Source: CAD feature listing. Evaluate the final solid. Frame: model axes, mm. Face numbers are marked on the shaded views. A direction names the side the tool comes from. Give positions to 0.01 mm unless a question says otherwise; leave off trailing zeros. Order: outer loops, then holes, each group sorted by start corner. A loop starts at its lowest first (then second) coordinate and runs counter-clockwise, first axis right, second up.
1) Section A-A, the plane z = 4.5. Return loops of the section in (x, y), plus the area to 3 significant figures.
2) Section D-D, the plane y = 30. Return loops of the section in (x, z), plus the area to 4 significant figures.
3) Section C-C, the plane x = -8. Return loops of the section in (y, z), plus the area to 3 significant figures.
4) Access query for the marked faces 1 and 2. Directions: +Z, -Z, +X, -X, +Y, -Y. A direction counts if a zero-diameter tool reaches every point of the face in a straight line with its end or side. Return the directions, or none.
5) Material intervals for line 1 (Y direction, x = 1, z = 0.25); line 2 (X direction, y = 25.5, z = -6.25); line 3 (Y direction, x = -7.75, z = 6.25), sorted ascending.
6) Draft query along Z for the marked faces 3, 4 and 5. Return one class per face: released by +Z, released by -Z, zero draft, split by the parting line, or undercut.
7) Section B-B, the plane x = 0.25. Return loops of the section in (y, z), plus the area to 3 significant figures.
8) First-contact query: P1, Ø2, axis at x = 0.5, z = -3.5, coming from the +Y side; P2, Ø13, axis at x = 3.5, y = 35, coming from the +Z side; P3, Ø2, axis at x = 4.5, z = 2, coming from the +Y side. Flat tips, straight axial feed; report the tip coordinate or a pass-through.
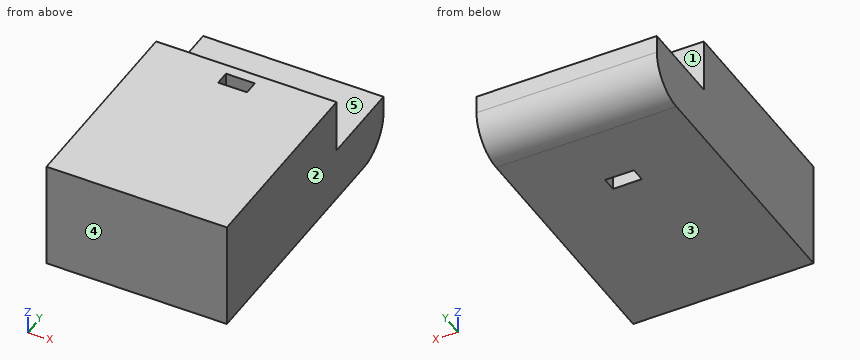
```python
from build123d import *

# Parameters (mm, degrees)
SKIZZE1_W                       = 25
SKIZZE1_H                       = 15
AUFSATZ_LINEAR_AUSTRAGEN1_DEPTH = 40
SKIZZE2_W                       = 25
SKIZZE2_H                       = 7.5
SCHNITT_LINEAR_AUSTRAGEN1_DEPTH = 12
VERRUNDUNG1_R                   = 5
SKIZZE3_W                       = 4
SKIZZE3_H                       = 2
SCHNITT_LINEAR_AUSTRAGEN2_DEPTH = 45.511234537


with BuildPart() as part:
    # Skizze1 → Aufsatz-Linear austragen1 (new body)
    with BuildSketch(Plane(origin=(0, 0, 0), x_dir=(1, 0, 0), z_dir=(0, 1, 0))):
        Rectangle(SKIZZE1_W, SKIZZE1_H)
    extrude(amount=AUFSATZ_LINEAR_AUSTRAGEN1_DEPTH)

    # Skizze2 → Schnitt-Linear austragen1 (cut)
    with BuildSketch(Plane(origin=(0, 40, 0), x_dir=(1, 0, 0), z_dir=(0, 1, 0))):
        with Locations((0, -3.75)):
            Rectangle(SKIZZE2_W, SKIZZE2_H)
    extrude(amount=-SCHNITT_LINEAR_AUSTRAGEN1_DEPTH, mode=Mode.SUBTRACT)

    # Verrundung1
    verrundung1_edges = [part.edges().sort_by_distance(p)[0] for p in [
        (0, 40, -7.5),
    ]]
    fillet(verrundung1_edges, radius=VERRUNDUNG1_R)

    # Skizze3 → Schnitt-Linear austragen2 (cut, through all)
    with BuildSketch(Plane.XY.offset(7.5)):
        with Locations((0, 25.494720236)):
            Rectangle(SKIZZE3_W, SKIZZE3_H)
    extrude(amount=-SCHNITT_LINEAR_AUSTRAGEN2_DEPTH, mode=Mode.SUBTRACT)


solid = part.part
```
From the geometry:
1. outline: (-12.5, 0) - (12.5, 0) - (12.5, 28) - (-12.5, 28) - close; hole (-2, 24.49) - (2, 24.49) - (2, 26.49) - (-2, 26.49) - close
1. area: 692 mm2
2. outline: (-12.5, -7.5) - (12.5, -7.5) - (12.5, 0) - (-12.5, 0) - close
2. area: 187.5 mm2
3. outline: (0, -7.5) - (35, -7.5) arc R5 ccw to (40, -2.5) - (40, 0) - (28, 0) - (28, 7.5) - (0, 7.5) - close
3. area: 505 mm2
4. face 1: +Z, +X, -X, +Y
4. face 2: +Z, -Z, +X, +Y, -Y
5. line 1: y = 0 to 24.49, 26.49 to 28
5. line 2: x = -12.5 to -2, 2 to 12.5
5. line 3: y = 0 to 28
6. face 3: released by -Z
6. face 4: zero draft
6. face 5: released by +Z
7. outline: (0, -7.5) - (24.49, -7.5) - (24.49, 7.5) - (0, 7.5) - close; (26.49, -7.5) - (35, -7.5) arc R5 ccw to (40, -2.5) - (40, 0) - (28, 0) - (28, 7.5) - (26.49, 7.5) - close
7. area: 475 mm2
8. P1: stops at y = 40
8. P2: stops at z = 0
8. P3: stops at y = 28
